Read the model definition and answer for the solid it produces. Units are mm, in the model's axes. A direction names the side the tool comes from. Round coordinates to 2 decimals unless told otherwise and drop trailing zeros. Order: outer loops, then holes, each group sorted by start corner. A loop starts at its lowest first (then second) coordinate and runs counter-clockwise, first axis right, second up.
from build123d import *


with BuildPart() as f1:
    # F0 (on Right) → F1 (revolve)
    with BuildSketch(Plane.YZ):
        Polygon((0, 6.5405), (0, 0), (5.08, 0), (5.08, 6.8961), (4.323409, 6.900981), (2.4892, 5.842), (1.524, 5.842), (1.524, 6.5405), align=None)
        Polygon((5.08, 6.8961), (5.08, 0), (32.639, 0), (32.639, 6.7183), align=None)
    revolve(axis=Axis((0, 18.390228, 0), (0, -1, 0)))

    # F2 (on Right) → F3 (revolve)
    with BuildSketch(Plane.YZ):
        with BuildLine():
            ThreePointArc((40.513, 3.592921), (36.774285, 5.545277), (32.639, 6.3754))
            Line((32.639, 6.3754), (32.639, 0))
            Line((32.639, 0), (40.513, 0))
            Line((40.513, 0), (40.513, 3.592921))
        make_face()
    revolve(axis=Axis((0, 36.576, 0), (0, -1, 0)))


solid = f1.part
Q1. Straight lines are drawn through the part: probe 1 along X at (y, z) = (13, 1.25); probe 2 along Z at (x, y) = (-2.25, 36); probe 3 along Y at (x, z) = (-4.5, 2.75). For each, find the intervals that lie inside material, in ascending order.
Outcome:
probe 1: x = -6.73 to 6.73
probe 2: z = -5.34 to 5.34
probe 3: y = 0 to 37.48
Q2. Flat-ended cylindrical pins translate along their axes: pin 1 (5 mm diameter, centred on x = 3, y = 7, fed in from +Z); pin 2 (4 mm diameter, centred on y = 25, z = -5.5, fed in from +X); pin 3 (5 mm diameter, centred on x = -1, y = 30, fed in from -Z). Find the tip coordinate at first contact, or state that the pin passes through.
Outcome:
pin 1: stops at z = 6.87
pin 2: stops at x = 5.79
pin 3: stops at z = -6.75
Q3. A cutting plane is placed at B-B, the plane y = 3. Give the vertices of the cut face in (x, z).
Outcome:
outline: circle Ø12.27 at (0, 0)
Q4. A cutting plane is placed at A-A, the plane y = 11.5. Give the vertices of the cut face in (x, z), plus the area to 3 significant figures.
Outcome:
outline: circle Ø13.71 at (0, 0)
area: 148 mm2
Q5. For a pull along Y with two mould halves and no side action, classify faces 3 (the face through (-6.485, 0.751, -0.851)), 4 (the face through (5.703, 2, -1.266)), 5 (the face through (0, 40.513, 0)) as released by +Y, released by -Y, zero draft, split by the parting line, or undercut.
Outcome:
face 3: zero draft
face 4: undercut
face 5: released by +Y
Q6. For faces 1 (the face through (-6, 1.524, 0)), 2 (the face through (0, 0, 0)), determine the directions among +Z, -Z, +X, -X, +Y, -Y from which every point of the face is accessible in a straight line to the end or side of a thin tool.
Outcome:
face 1: none
face 2: +Z, -Z, +X, -X, -Y
